Read the model definition and answer for the solid it produces. Units are mm, in the model's axes. Face numbers are marked on the shaded views. A direction names the side the tool comes from. Round coordinates to 2 decimals unless told otherwise and drop trailing zeros. Write each loop counter-clockwise with the first axis right and the second up, starting at its lowest first coordinate (ties: lowest second). Pieces come first, ordered by that corner, then holes.
from build123d import *

# Parameters (mm, degrees)
SZKIC1_W                    = 8
SZKIC1_H                    = 45
DODANIE_WYCI_GNI_CIE1_DEPTH = 7
SZKIC2_R                    = 1.05
WYTNIJ_WYCI_GNI_CIE1_DEPTH  = 7
SZKIC3_W                    = 2
SZKIC3_H                    = 37
WYTNIJ_WYCI_GNI_CIE2_DEPTH  = 0.5
SZKIC4_W                    = 2
SZKIC4_H                    = 5
DODANIE_WYCI_GNI_CIE4_DEPTH = 5
SZKIC13_R                   = 0.75
DODANIE_WYCI_GNI_CIE7_DEPTH = 3.5
ZAOKR_GLENIE1_R             = 0.8
SZKIC14_W                   = 2
SZKIC14_H                   = 1
WYTNIJ_WYCI_GNI_CIE3_DEPTH  = 1


with BuildPart() as part:
    # Szkic1 → Dodanie-wyciągnięcie1 (new body)
    with BuildSketch(Plane(origin=(0, 0, 0), x_dir=(1, 0, 0), z_dir=(0, 1, 0))):
        with Locations((4, 22.5)):
            Rectangle(SZKIC1_W, SZKIC1_H)
    extrude(amount=DODANIE_WYCI_GNI_CIE1_DEPTH)

    # Szkic2 → Wytnij-wyciągnięcie1 (cut)
    with BuildSketch(Plane(origin=(0, 7, 0), x_dir=(1, 0, 0), z_dir=(0, 1, 0))):
        with Locations((4, 2)):
            Circle(SZKIC2_R)
        with Locations((4, 43)):
            Circle(SZKIC2_R)
    extrude(amount=-WYTNIJ_WYCI_GNI_CIE1_DEPTH, mode=Mode.SUBTRACT)

    # Szkic3 → Wytnij-wyciągnięcie2 (cut)
    with BuildSketch(Plane(origin=(0, 7, 0), x_dir=(1, 0, 0), z_dir=(0, 1, 0))):
        with Locations((4, 22.5)):
            Rectangle(SZKIC3_W, SZKIC3_H)
    extrude(amount=-WYTNIJ_WYCI_GNI_CIE2_DEPTH, mode=Mode.SUBTRACT)

    # Szkic4 → Dodanie-wyciągnięcie4 (add)
    with BuildSketch(Plane(origin=(0, 6.5, 0), x_dir=(1, 0, 0), z_dir=(0, 1, 0))):
        with Locations((4, 7.3)):
            Rectangle(SZKIC4_W, SZKIC4_H)
    extrude(amount=DODANIE_WYCI_GNI_CIE4_DEPTH)

    # Szkic13 → Dodanie-wyciągnięcie7 (add)
    with BuildSketch(Plane.XZ):
        with Locations((2.125, -40)):
            Circle(SZKIC13_R)
        with Locations((5.875, -40)):
            Circle(SZKIC13_R)
        with Locations((2.125, -5)):
            Circle(SZKIC13_R)
    extrude(amount=DODANIE_WYCI_GNI_CIE7_DEPTH)

    # Zaokrąglenie1
    zaokr_glenie1_edges = [part.edges().sort_by_distance(p)[0] for p in [
        (0, 3.5, -45),
        (8, 3.5, -45),
        (8, 3.5, 0),
        (0, 3.5, 0),
    ]]
    fillet(zaokr_glenie1_edges, radius=ZAOKR_GLENIE1_R)

    # Szkic14 → Wytnij-wyciągnięcie3 (cut)
    with BuildSketch(Plane(origin=(0, 11.5, 0), x_dir=(1, 0, 0), z_dir=(0, 1, 0))):
        with Locations((4, 7.3)):
            Rectangle(SZKIC14_W, SZKIC14_H)
    extrude(amount=-WYTNIJ_WYCI_GNI_CIE3_DEPTH, mode=Mode.SUBTRACT)


solid = part.part
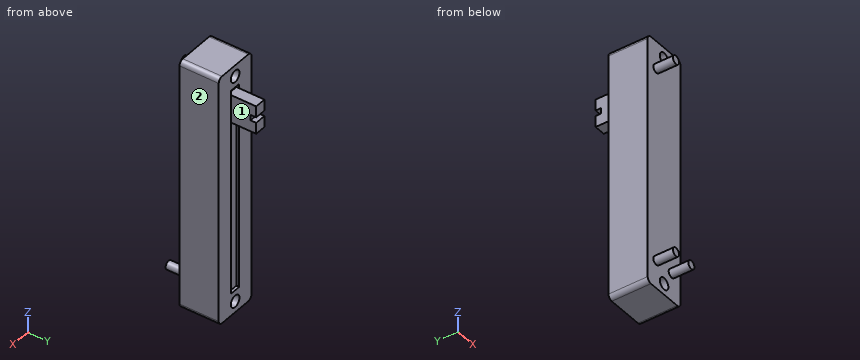
Q1. Straight lines are drawn through the part: probe 1 along Z at (x, y) = (4, 2.25); probe 2 along X at (y, z) = (4.25, -43); probe 3 along Y at (x, z) = (4.5, -29). For each, find the intervals that lie inside material, in ascending order.
Verdict:
probe 1: z = -45 to -44.05, -41.95 to -3.05, -0.95 to 0
probe 2: x = 0 to 2.95, 5.05 to 8
probe 3: y = 0 to 6.5
Q2. Section C-C (y = 4.75) is taken. Determine the outline of the cut face in (x, z).
Verdict:
outline: (0, -44.2) arc R0.8 ccw to (0.8, -45) - (7.2, -45) arc R0.8 ccw to (8, -44.2) - (8, -0.8) arc R0.8 ccw to (7.2, 0) - (0.8, 0) arc R0.8 ccw to (0, -0.8) - close; hole circle Ø2.1 at (4, -43); hole circle Ø2.1 at (4, -2)
Q3. Which of the six approach directions +Z, -Z, +X, -X, +Y, -Y give full straight-line access (tool end or side, diameter ignored) to the marked faces 1 and 2?
Verdict:
face 1: +Z, -Z, +X, +Y
face 2: +Z, -Z, +X, +Y, -Y
Q4. Section B-B (z = -43) is taken. Determine the outline of the cut face in (x, y).
Verdict:
outline: (0, 0) - (2.95, 0) - (2.95, 7) - (0, 7) - close; (5.05, 0) - (8, 0) - (8, 7) - (5.05, 7) - close
Q5. Flat-ended cylindrical pins translate along their axes: pin 1 Ø0.6 at (x, y) = (4, 9) entering from -Z; pin 2 Ø4 at (x, z) = (4.5, -15.5) entering from -Y; pin 3 Ø1 at (x, y) = (3.5, 9.5) entering from +Z. Find the tip coordinate at first contact, or state that the pin passes through.
Verdict:
pin 1: stops at z = -9.8
pin 2: stops at y = 0
pin 3: stops at z = -4.8
Q6. Section A-A (x = 4) is taken. Determine the outline of the cut face in (y, z), then the cut area to 3 significant figures.
Verdict:
outline: (0, -45) - (7, -45) - (7, -44.05) - (0, -44.05) - close; (0, -41.95) - (7, -41.95) - (7, -41) - (6.5, -41) - (6.5, -9.8) - (11.5, -9.8) - (11.5, -7.8) - (10.5, -7.8) - (10.5, -6.8) - (11.5, -6.8) - (11.5, -4.8) - (6.5, -4.8) - (6.5, -4) - (7, -4) - (7, -3.05) - (0, -3.05) - close; (0, -0.95) - (7, -0.95) - (7, 0) - (0, 0) - close
area: 291 mm2
Q7. Section D-D (y = -1.5) is taken. Determine the outline of the cut face in (x, z) (3 decimals), then the cut area to 3 significant figures.
Verdict:
outline: circle Ø1.5 at (2.125, -40); circle Ø1.5 at (2.125, -5); circle Ø1.5 at (5.875, -40)
area: 5.30 mm2
